from build123d import *

# Parameters (mm, degrees)
SKETCH_1_R          = 50
SKETCH_1_R_2        = 1.65
SKETCH_1_W          = 43
SKETCH_1_H          = 43
EXTRUDE_1_DEPTH     = 4
SKETCH_2_R          = 3.15
CUT_EXTRUDE_1_DEPTH = 2
FILLET_1_R          = 4


with BuildPart() as part:
    # 草图1 → 凸台-拉伸1 (new body)
    with BuildSketch(Plane.XY):
        Circle(SKETCH_1_R)
        with Locations((-38.97114317, 22.5)):
            Circle(SKETCH_1_R_2, mode=Mode.SUBTRACT)
        with Locations((0, 45)):
            Circle(SKETCH_1_R_2, mode=Mode.SUBTRACT)
        with Locations((38.97114317, 22.5)):
            Circle(SKETCH_1_R_2, mode=Mode.SUBTRACT)
        with Locations((38.97114317, -22.5)):
            Circle(SKETCH_1_R_2, mode=Mode.SUBTRACT)
        with Locations((0, -45)):
            Circle(SKETCH_1_R_2, mode=Mode.SUBTRACT)
        with Locations((-38.97114317, -22.5)):
            Circle(SKETCH_1_R_2, mode=Mode.SUBTRACT)
        Rectangle(SKETCH_1_W, SKETCH_1_H, mode=Mode.SUBTRACT)
    extrude(amount=EXTRUDE_1_DEPTH)

    # 草图2 → 切除-拉伸1 (cut)
    with BuildSketch(Plane.XY):
        with Locations((0, 45)):
            Circle(SKETCH_2_R)
        with Locations((38.97114317, 22.5)):
            Circle(SKETCH_2_R)
        with Locations((38.97114317, -22.5)):
            Circle(SKETCH_2_R)
        with Locations((0, -45)):
            Circle(SKETCH_2_R)
        with Locations((-38.97114317, -22.5)):
            Circle(SKETCH_2_R)
        with Locations((-38.97114317, 22.5)):
            Circle(SKETCH_2_R)
    extrude(amount=CUT_EXTRUDE_1_DEPTH, mode=Mode.SUBTRACT)

    # 圆角1
    fillet_1_edges = [part.edges().sort_by_distance(p)[0] for p in [
        (21.5, -21.5, 2),
        (21.5, 21.5, 2),
        (-21.5, 21.5, 2),
        (-21.5, -21.5, 2),
    ]]
    fillet(fillet_1_edges, radius=FILLET_1_R)


solid = part.part
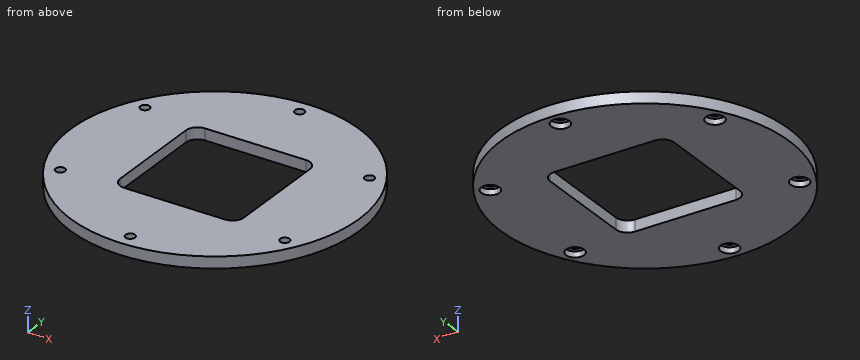
CAD build for the part. Positions are in the model's coordinates, mm. Give positions to 0.01 mm unless a question says otherwise; leave off trailing zeros. Loops run counter-clockwise (first coordinate to the right, second up) from the corner with the lowest first, then second, coordinate; pieces in that order, holes last. Notation, with made-up numbers: M 68.5,59.25 L 111.5,59.25 A19 ccw 111.5,76.25 Z; hole C 7,58 d11. An arc over 180 degrees is marked long. One line per question, with ' | ' between items. Start each with the question number.
1. Probe L1, parallel to Y at x = 0, z = 0.9; L2, parallel to X at y = 24, z = 2.95; L3, parallel to X at y = -19, z = 3.8. List the from-to ranges inside material, lowest first. Write a range as from..to.
2. Flat gauge pins, fed straight in: pin 1 (1 mm diameter, centred on x = 28, z = 1.5, fed in from -Y); pin 2 (2 mm diameter, centred on x = -38.97, y = 22.5, fed in from +Z); pin 3 (3 mm diameter, centred on x = 0.5, y = -45, fed in from -Z); pin 4 (1 mm diameter, centred on y = -26, z = 3.5, fed in from -X). Where does each tip first touch, or does it go through?
3. Saw through at B-B on z = 3.4. Give the cut face in (x, y).
4. Saw through at A-A on x = 0. Give the cut face in (y, z), plus the area to 3 significant figures.
5. Saw through at C-C on y = 45. Give the cut face in (x, z), plus the area to 3 significant figures.
6. Saw through at D-D on y = -32.5. Give the cut face in (x, z), plus the area to 3 significant figures.
Result sheet:
1) L1: y = -50..-48.15, -41.85..-21.5, 21.5..41.85, 48.15..50 | L2: x = -43.86..-39.66, -38.28..38.28, 39.66..43.86 | L3: x = -46.25..-21.21, 21.21..46.25
2) pin 1: stops at y = -41.76 | pin 2: passes through | pin 3: stops at z = 2 | pin 4: stops at x = -43.01
3) outline: C 0,0 d100; hole C -38.97,-22.5 d3.3; hole C -38.97,22.5 d3.3; hole M -21.5,-17.5 A4 ccw -17.5,-21.5 L 17.5,-21.5 A4 ccw 21.5,-17.5 L 21.5,17.5 A4 ccw 17.5,21.5 L -17.5,21.5 A4 ccw -21.5,17.5 Z; hole C 0,-45 d3.3; hole C 0,45 d3.3; hole C 38.97,-22.5 d3.3; hole C 38.97,22.5 d3.3
4) outline: M -50,0 L -48.15,0 L -48.15,2 L -46.65,2 L -46.65,4 L -50,4 Z; M -43.35,2 L -41.85,2 L -41.85,0 L -21.5,0 L -21.5,4 L -43.35,4 Z; M 21.5,0 L 41.85,0 L 41.85,2 L 43.35,2 L 43.35,4 L 21.5,4 Z; M 46.65,2 L 48.15,2 L 48.15,0 L 50,0 L 50,4 L 46.65,4 Z | area: 190 mm^2
5) outline: M -21.79,0 L -3.15,0 L -3.15,2 L -1.65,2 L -1.65,4 L -21.79,4 Z; M 1.65,2 L 3.15,2 L 3.15,0 L 21.79,0 L 21.79,4 L 1.65,4 Z | area: 155 mm^2
6) outline: M -38,0 L 38,0 L 38,4 L -38,4 Z | area: 304 mm^2
